CAD build for the part. Positions are in the model's coordinates, mm. A direction names the side the tool comes from. Round coordinates to 2 decimals unless told otherwise and drop trailing zeros. Loops run counter-clockwise (first coordinate to the right, second up) from the corner with the lowest first, then second, coordinate; pieces in that order, holes last. Notation, with made-up numbers: M 13.5,-12.75 L 18.5,-12.75 A31 cw 18.5,11.25 Z; hole C -2.75,58.25 d5. An arc over 180 degrees is marked long. Put each result on its own line as item: value. Start each with the question number.
Autodesk Inventor part; units mm, degrees
ref_plane "YZ Plane" through (0, 0, 0) normal (1, 0, 0) x (0, 1, 0)
ref_plane "XZ Plane" through (0, 0, 0) normal (0, 1, 0) x (-1, 0, 0)
ref_plane "XY Plane" through (0, 0, 0) normal (0, 0, 1) x (1, 0, 0)
sketch "Sketch1" plane through (0, 0, 0) normal (0, 0, 1) x (1, 0, 0)
  line L0 (-15.875, 0) -> (15.875, 0)
  line L1 (15.875, 0) -> (15.875, 38.1)
  line L2 (15.875, 38.1) -> (-15.875, 38.1)
  line L3 (-15.875, 38.1) -> (-15.875, 0)
  point P0 (0, 0)
  dimension "d2" = 31.75
  dimension "d3" = 38.1
  dimension "d4" = 15.875
  dimension "d5" = 0
extrude "Extrusion1" add sketch "Sketch1" along normal blind 139.7
sketch "Sketch2" plane through (0, 0, 139.7) normal (0, 0, 1) x (1, 0, 0)
  arc A0 (-12.065, 19.05) -> (12.065, 19.05) centre (0, 19.05) ccw
  line L0 (-15.875, 0) -> (15.875, 0)
  line L1 (12.065, 19.05) -> (12.065, 38.1)
  line L2 (15.875, 38.1) -> (-15.875, 38.1)
  line L3 (-12.065, 19.05) -> (-12.065, 38.1)
  point P0 (0, 0)
  dimension "d8" = 19.05
  dimension "d9" = 24.13
extrude "Extrusion2" cut sketch "Sketch2" against normal through all
sketch "Sketch3" plane through (-15.875, 0, 0) normal (0, -1, 0) x (1, 0, 0)
  circle A0 centre (28.575, 8.89) radius 2
  circle A1 centre (3.175, 130.81) radius 2
  line L0 (15.875, 0) -> (15.875, 139.7) construction
  line L1 (0, 139.7) -> (31.75, 139.7) construction
  line L2 (0, 0) -> (31.75, 0) construction
  line L3 (31.75, 139.7) -> (0, 139.7) construction
  circle A2 centre (28.575, 111.76) radius 2
  line L4 (31.75, 0) -> (31.75, 139.7)
  dimension "d12" = 4
  dimension "d13" = 4
  dimension "d14" = 12.7
  dimension "d15" = 8.89
  dimension "d16" = 12.7
  dimension "d17" = 8.89
  dimension "d28" = 4
  dimension "d30" = 27.94
  dimension "d32" = 12.7
extrude "Heat Set Inserts" cut sketch "Sketch3" against normal blind 7
sketch "Sketch4" plane through (0, 0, 139.7) normal (0, 0, 1) x (1, 0, 0)
  line L0 (-15.875, 0) -> (15.875, 0)
  line L1 (15.875, 0) -> (15.875, 38.1)
  line L2 (-15.875, 0) -> (15.875, 0)
  line L3 (15.875, 0) -> (15.875, 19.05)
  line L4 (15.875, 19.05) -> (-15.875, 19.05)
  line L5 (-15.875, 19.05) -> (-15.875, 0)
  point P0 (0, 0)
  dimension "d20" = 19.05
extrude "Back Wall" add sketch "Sketch4" along normal blind 1.5875
sketch "Sketch5" plane through (0, 0, 0) normal (0, 0, -1) x (-1, 0, 0)
  line L0 (15.875, 0) -> (-15.875, 0)
  line L1 (15.875, 19.05) -> (15.875, 0)
  line L2 (-15.875, 0) -> (15.875, 0)
  line L3 (15.875, 0) -> (15.875, 10.16)
  line L4 (15.875, 10.16) -> (-15.875, 10.16)
  line L5 (-15.875, 10.16) -> (-15.875, 0)
  point P0 (0, 0)
  dimension "d23" = 10.16
extrude "Extrusion5" add sketch "Sketch5" along normal blind 1.5875
sketch "Sketch6" plane through (0, 0, -1.5875) normal (0, 0, -1) x (-1, 0, 0)
  line L0 (15.875, 0) -> (-15.875, 0)
  line L1 (-15.875, 38.1) -> (15.875, 38.1)
  line L2 (15.875, 38.1) -> (15.875, 0)
  line L3 (15.875, 0) -> (-15.875, 0)
  line L4 (-15.875, 0) -> (-15.875, 38.1)
  point P0 (0, 0)
extrude "Extrusion6" cut sketch "Sketch6" against normal blind 101.6
equation "\"d12\" = m3_heat_set_insert"
equation "\"d13\" = m3_heat_set_insert"
equation "\"d28\" = d29"
equation "\"d32\" = d16"
equation "\"d18\" = m3_heat_set_depth"
equation "\"m3_heat_set_insert\" = 4"
equation "\"m3_clearance\" = 3.4"
equation "\"m3_heat_set_depth\" = 7"
equation "\"robot_diameter\" = 354"
equation "\"hardboard_thickness\" = 5"
properties part number "NiMH_Holder_Back"
(1) Tool access for faces 1 (the cylindrical face through (-0.27, 6.99, 120.13)), 2 (the flat face through (0, 19.05, 140)), 3 (the cylindrical face through (12.3, 3.5, 109.8)): list every direction of +Z, -Z, +X, -X, +Y, -Y with a clear straight run to the whole face (end or side of a thin tool).
(2) Cut at D-D on y = 16.5. List the corners of the cut face in (x, z) (1 decimal).
(3) Cut at C-C on x = 12.7. List the corners of the cut face in (y, z).
(4) Flat gauge pins, fed straight in: pin 1 Ø1.3 at (x, z) = (-2, 140) entering from +Y; pin 2 Ø3 at (x, y) = (14.5, 26.5) entering from +Z; pin 3 Ø2 at (x, z) = (-13, 131.5) entering from -Y. Where does each tip first touch, or does it go through?
(5) Cut at A-A on y = 23.5. List the corners of the cut face in (x, z) (1 decimal).
(6) Mould opens along X. For faces 4 (the flat face through (-12.065, 28, 120)), 5 (the flat face through (-14, 29, 139.7)), 6 (the flat face through (15.875, 19, 121)) say: +X half, -X half, draft (parallel to the pull), parting line (faces both ways), or undercut.
(7) Drill centre lines: line 1 along X through (y, z) = (28.5, 134) (3 decimals); line 2 along X through (y, z) = (3, 130.81) (3 decimals); line 3 along Z through (x, y) = (-12.7, 3.25). Where is each one in solid material? Low to high.
(8) Cut at B-B on z = 130.81. List the corners of the cut face in (x, y) (3 decimals).
Taken from the geometry:
1. face 1: -Z, +Y
1. face 2: +Z, +X, -X, +Y
1. face 3: -Y
2. outline: M -15.9,100 L -11.8,100 L -11.8,139.7 L 11.8,139.7 L 11.8,100 L 15.9,100 L 15.9,141.3 L -15.9,141.3 Z
3. outline: M 0,100.01 L 38.1,100.01 L 38.1,139.7 L 19.05,139.7 L 19.05,141.29 L 0,141.29 L 0,113.76 L 7,113.76 L 7,109.76 L 0,109.76 Z
4. pin 1: y = 19.05
4. pin 2: z = 139.7
4. pin 3: y = 7
5. outline: M -15.9,100 L -12.1,100 L -12.1,139.7 L -15.9,139.7 Z; M 12.1,100 L 15.9,100 L 15.9,139.7 L 12.1,139.7 Z
6. face 4: undercut
6. face 5: draft
6. face 6: +X half
7. line 1: -15.875 to -12.065, 12.065 to 15.875
7. line 2: -15.875 to -14.7, -10.7 to 15.875
7. line 3: 100.01 to 128.81, 132.81 to 141.29
8. outline: M -15.875,0 L -14.7,0 L -14.7,7 L -10.7,7 L -10.7,0 L 15.875,0 L 15.875,38.1 L 12.065,38.1 L 12.065,19.05 A12.065 cw -12.065,19.05 L -12.065,38.1 L -15.875,38.1 Z
